from build123d import *

# Parameters (mm, degrees)
F0_W      = 76.2
F0_H      = 25.4
F1_DEPTH  = 101.6
F0_H_2    = 76.2
F2_DEPTH  = 25.4
F4_DEPTH  = 101.601
F7_DEPTH  = 25.401
F9_R      = 12.7
F8_R      = 12.7
F10_DEPTH = 25.401


with BuildPart() as f1:
    # F0 (on Top) → F1 (new body)
    with BuildSketch(Plane.XY):
        Polygon((68.37053, 61.854359), (42.97053, 61.854359), (42.97053, -14.345641), (42.97053, -39.745641), (42.97053, -115.945641), (68.37053, -115.945641), align=None)
        with Locations((4.87053, -27.045641)):
            Rectangle(F0_W, F0_H)
    extrude(amount=F1_DEPTH)

    # F0 (on Top) → F2 (join)
    with BuildSketch(Plane.XY):
        with Locations((4.87053, 23.754359)):
            Rectangle(F0_W, F0_H_2)
        with Locations((4.87053, -77.845641)):
            Rectangle(F0_W, F0_H_2)
    extrude(amount=F2_DEPTH)

    # F3 (on face) → F4 (cut, through all)
    with BuildSketch(Plane.XZ.offset(39.745641)):
        Polygon((-33.22947, 101.6), (-33.22947, 25.4), (42.97053, 101.6), align=None)
    extrude(amount=-F4_DEPTH, mode=Mode.SUBTRACT)

    # F6 (on face) + F5 (on face) → F7 (cut, through all)
    with BuildSketch(Plane(origin=(42.97053, 0, 0), x_dir=(0, -1, 0), z_dir=(-1, 0, 0))):
        Polygon((-61.854359, 63.5), (-23.754359, 101.6), (-61.854359, 101.6), align=None)
    with BuildSketch(Plane(origin=(42.97053, 0, 0), x_dir=(0, -1, 0), z_dir=(-1, 0, 0))):
        Polygon((115.945641, 101.6), (77.845641, 101.6), (115.945641, 63.5), align=None)
    extrude(amount=-F7_DEPTH, mode=Mode.SUBTRACT)

    # F9 (on face) + F8 (on face) → F10 (cut, through all)
    with BuildSketch(Plane.XY.offset(25.4)):
        with Locations((4.87053, 23.754359)):
            Circle(F9_R)
    with BuildSketch(Plane.XY.offset(25.4)):
        with Locations((4.87053, -77.845641)):
            Circle(F8_R)
    extrude(amount=-F10_DEPTH, mode=Mode.SUBTRACT)


solid = f1.part
The model under review builds one solid part; all positions refer to its coordinate system, in mm. A direction names the side the tool comes from. Give positions to 0.01 mm unless a question says otherwise; leave off trailing zeros. Loops run counter-clockwise (first coordinate to the right, second up) from the corner with the lowest first, then second, coordinate; pieces in that order, holes last. Notation, with made-up numbers: (56.25, 3.25) -> (102.25, 3.25) arc R16 cw to (102.25, 9.25) -> close; hole circle Ø9 at (69, 64.25). An arc over 180 degrees is marked (long way). Answer as a JSON object with one key per item and string values. Group by question number.
Q1. Tool access review of faces 4 (the flat face through (21, -39.746, 46)), 5 (the flat face through (42.971, 24, 63)), 6 (the flat face through (28, -115.946, 17)): name each direction out of +Z, -Z, +X, -X, +Y, -Y from which nothing blocks a thin tool from reaching the whole face with its end or side.
Q2. Insertion check: pin 1 (23 mm diameter, centred on x = 9, z = 56.5, fed in from +Y); pin 2 (10 mm diameter, centred on x = 14, y = -88.5, fed in from -Z); pin 3 (12 mm diameter, centred on x = 29, z = 32.5, fed in from -Y); pin 4 (3 mm diameter, centred on x = -17.5, y = -43.5, fed in from +Z). Each pin has a flat end and moves straight along its axis. Give the tip position at first contact, or say it passes through.
Q3. Take a section at A-A (x = 9). Write out the cut boundary in (y, z).
Q4. Take a section at C-C (y = -86.5). Write out the cut boundary in (x, z), plus the area to 3 significant figures.
Q5. Wall thickness on line 1 along Z through (x, y) = (-0.5, -94); line 2 along X through (y, z) = (-84, 6.5); line 3 along X through (y, z) = (-3, 93.5): over which ranges is each line inside the solid? List them lowest first.
Q6. Draft analysis for pull direction Y (two halves, no side actions). For faces 1 (the cylindrical face through (11.7, 34.46, 12.88)), 2 (the flat face through (21, -14.346, 46)), 3 (the flat face through (-13, -77, 25.4)), state which applies: pulls with the +Y half, pulls with the -Y half, needs draft (parallel to the pull), parting line crosses it, or undercut.
Q7. Take a section at D-D (z = 90). Write out the cut boundary in (x, y).
Q8. Take a section at B-B (z = 14). Write out the cut boundary in (x, y), plus the area to 3 significant figures.
Answer below:
{
 "1": {"face 4": "+Z, -X, -Y", "face 5": "+Z, -X, +Y", "face 6": "+Z, -Z, +X, -X, -Y"},
 "2": {"pin 1": "stops at y = -14.35", "pin 2": "stops at z = 0", "pin 3": "stops at y = -39.75", "pin 4": "stops at z = 25.4"},
 "3": {"outline": "(-115.95, 0) -> (-89.86, 0) -> (-89.86, 25.4) -> (-115.95, 25.4) -> close; (-65.84, 0) -> (11.74, 0) -> (11.74, 25.4) -> (-14.35, 25.4) -> (-14.35, 67.63) -> (-39.75, 67.63) -> (-39.75, 25.4) -> (-65.84, 25.4) -> close; (35.76, 0) -> (61.85, 0) -> (61.85, 25.4) -> (35.76, 25.4) -> close"},
 "4": {"outline": "(-33.23, 0) -> (-4.42, 0) -> (-4.42, 25.4) -> (-33.23, 25.4) -> close; (14.17, 0) -> (68.37, 0) -> (68.37, 92.95) -> (42.97, 92.95) -> (42.97, 25.4) -> (14.17, 25.4) -> close", "area": "3,820 mm2"},
 "5": {"line 1": "z = 0 to 25.4", "line 2": "x = -33.23 to -6.24, 15.98 to 68.37", "line 3": "x = 42.97 to 68.37"},
 "6": {"face 1": "undercut", "face 2": "pulls with the +Y half", "face 3": "needs draft"},
 "7": {"outline": "(31.37, -39.75) -> (42.97, -39.75) -> (42.97, -89.45) -> (68.37, -89.45) -> (68.37, 35.35) -> (42.97, 35.35) -> (42.97, -14.35) -> (31.37, -14.35) -> close"},
 "8": {"outline": "(-33.23, -115.95) -> (68.37, -115.95) -> (68.37, 61.85) -> (-33.23, 61.85) -> close; hole circle Ø25.4 at (4.87, -77.85); hole circle Ø25.4 at (4.87, 23.75)", "area": "17,100 mm2"}
}
